The model under review builds one solid part; all positions refer to its coordinate system, in mm. A direction names the side the tool comes from. Round coordinates to 2 decimals unless told otherwise and drop trailing zeros. Write each loop counter-clockwise with the first axis right and the second up, starting at its lowest first coordinate (ties: lowest second). Pieces come first, ordered by that corner, then holes.
Item 1: Add section D-D (z = 322.25). Give the boundary of the cut face in (x, y).
Item 2: Add section C-C (y = -6). Give the boundary of the cut face in (x, z).
Item 3: Machinability: for faces 4 (the face through (-24, -58, 290)), 5 (the face through (0, -17, 128)), 6 (the face through (-66, -2.5, 157)), which of the approach directions +Z, -Z, +X, -X, +Y, -Y give a long, thin tool a straight path to every point of the face, cutting with its end or side? Answer none if there is none.
Item 4: Add section B-B (z = 23). Give the boundary of the cut face in (x, y), plus the area to 3 significant figures.
Item 5: Draft analysis for pull direction Z (two halves, no side actions). For faces 1 (the face through (-66, -31, 310)), 2 (the face through (-127.5, -30, 153)), 3 (the face through (-66, -3, 317)), state which applies: +Z half, -Z half, draft (parallel to the pull), parting line (faces both ways), or undercut.
Item 6: To check wall thickness, follow L1, parallel to X at y = -13.5, z = 236; L2, parallel to Z at x = -18, y = -32.5; L3, parallel to Y at x = -101, z = 220.5. State the ranges of each line that lie inside material, in increasing order.
Item 7: Add section A-A (x = -65). Give the boundary of the cut face in (y, z), plus the area to 3 significant figures.
Item 8: Clearance check with flat-ended pins moving along their axes: pin 1 Ø12.5 at (x, z) = (-65.5, 326) entering from -Y; pin 2 Ø3 at (x, z) = (-1, 178) entering from -Y; pin 3 Ø0.8 at (y, z) = (-58, 185.5) entering from +X. State where each tip first meets the part, or that it passes through.
```python
from build123d import *

# Parameters (mm, degrees)
F0_W      = 130
F0_H      = 310
F1_DEPTH  = 60
F3_DEPTH  = 30
F4_T      = -2.5
F5_W      = 130
F5_H      = 3
F6_DEPTH  = 25
F10_DEPTH = 3.001
F11_DEPTH = 25
F12_DEPTH = 3.001


# Not quite as in the source:
# - a feature of the source that left no trace in its solid (it failed there, or was rolled back) is left out


with BuildPart() as f1:
    # F0 (on Front) → F1 (new body)
    with BuildSketch(Plane.XZ):
        with Locations((-65, 155)):
            Rectangle(F0_W, F0_H)
    extrude(amount=F1_DEPTH)

    # F2 (on face) → F3 (cut)
    with BuildSketch(Plane.XZ.offset(60)):
        Polygon((0, 50), (0, 290), (-70, 290), (-70, 50), (-48.1321327388, 50), align=None)
    extrude(amount=-F3_DEPTH, mode=Mode.SUBTRACT)

    # F4
    f4_openings = [f1.faces().sort_by_distance(p)[0] for p in [
        (-35, -45, 50),
        (-70, -45, 170),
        (-35, -30, 170),
        (-35, -45, 290),
    ]]
    offset(amount=F4_T, openings=f4_openings)

    # F5 (on face) → F6 (join)
    with BuildSketch(Plane.XY.offset(310)):
        with Locations((-65, -1.5)):
            Rectangle(F5_W, F5_H)
    extrude(amount=F6_DEPTH)

    # F9 (on face) → F10 (cut, through all)
    with BuildSketch(Plane.XZ.offset(3)):
        with BuildLine():
            Line((-50, 326), (-60, 326))
            ThreePointArc((-60, 326), (-65, 331), (-70, 326))
            Line((-70, 326), (-80, 326))
            ThreePointArc((-80, 326), (-83.75, 322.25), (-80, 318.5))
            Line((-80, 318.5), (-50, 318.5))
            ThreePointArc((-50, 318.5), (-46.25, 322.25), (-50, 326))
        make_face()
    extrude(amount=-F10_DEPTH, mode=Mode.SUBTRACT)

    # F5 (on face) → F11 (join)
    with BuildSketch(Plane.XY.offset(310)):
        with Locations((-65, -1.5)):
            Rectangle(F5_W, F5_H)
    extrude(amount=F11_DEPTH)

    # F9 (on face) → F12 (cut, through all)
    with BuildSketch(Plane.XZ.offset(3)):
        with BuildLine():
            Line((-50, 326), (-60, 326))
            ThreePointArc((-60, 326), (-65, 331), (-70, 326))
            Line((-70, 326), (-80, 326))
            ThreePointArc((-80, 326), (-83.75, 322.25), (-80, 318.5))
            Line((-80, 318.5), (-50, 318.5))
            ThreePointArc((-50, 318.5), (-46.25, 322.25), (-50, 326))
        make_face()
    extrude(amount=-F12_DEPTH, mode=Mode.SUBTRACT)


solid = f1.part
```
Numbers:
1. outline: (-130, -3) - (-83.75, -3) - (-83.75, 0) - (-130, 0) - close; (-46.25, -3) - (0, -3) - (0, 0) - (-46.25, 0) - close
2. outline: (-130, 0) - (0, 0) - (0, 310) - (-130, 310) - close; hole (-127.5, 2.5) - (-2.5, 2.5) - (-2.5, 307.5) - (-127.5, 307.5) - close
3. face 4: +X, -Y
3. face 5: +Z, -Z, +X, +Y, -Y
3. face 6: none
4. outline: (-130, -60) - (0, -60) - (0, 0) - (-130, 0) - close; hole (-127.5, -57.5) - (-2.5, -57.5) - (-2.5, -2.5) - (-127.5, -2.5) - close
4. area: 925 mm2
5. face 1: +Z half
5. face 2: undercut
5. face 3: draft
6. L1: x = -130 to -127.5, -2.5 to 0
6. L2: z = 0 to 2.5, 307.5 to 310
6. L3: y = -60 to -57.5, -2.5 to 0
7. outline: (-60, 0) - (0, 0) - (0, 318.5) - (-3, 318.5) - (-3, 310) - (-60, 310) - (-60, 290) - (-57.5, 290) - (-57.5, 307.5) - (-2.5, 307.5) - (-2.5, 2.5) - (-57.5, 2.5) - (-57.5, 50) - (-60, 50) - close; (-3, 331) - (0, 331) - (0, 335) - (-3, 335) - close
7. area: 1,260 mm2
8. pin 1: stops at y = -3
8. pin 2: stops at y = -30
8. pin 3: stops at x = -70
